The drawing under review shows one solid part. Ordinate dimensions are in mm from its lowest x, y, z. A direction names the side the tool comes from. Coordinates: 2 decimals unless noted, no trailing zeros. Write each loop counter-clockwise with the first axis right and the second up, starting at its lowest first coordinate (ties: lowest second). Pieces come first, ordered by that corner, then holes. Notation, with made-up numbers: (-30.75, -19.5) -> (25.25, -19.5) arc R12 cw to (25.25, -1.5) -> close; hole circle Ø10 at (26, 15). An arc over 180 degrees is marked (long way). One line per question, with ' | ' between items. Start each with the question number.
Q1. Add section C-C on z = 4.75. State the section outline as (x, y) points.
Q2. Wall thickness on probe 1 along X at (y, z) = (11, 5.55); probe 2 along X at (y, z) = (13, 1.9): over which ranges is each line inside the solid? List them lowest first.
Q3. For P1, Ø1.2, axis at x = 4.5, y = 24, coming from the +Z side; P2, Ø3, axis at y = 18, z = 4.5, coming from the +X side; P3, Ø2, axis at x = 2.5, y = 19, coming from the +Z side; P4, Ø1, axis at x = 1, y = 21, coming from the -Z side, all flat-tipped, find the tip position at first contact; note any pin that passes through.
Q4. Add section A-A on y = 31.5. State the section outline as (x, z) points, and give its area (3 significant figures).
Q5. For the marked faces 1 and 2, list the 3-axis set-ups (+Z, -Z, +X, -X, +Y, -Y) from which the entire face can be reached by the end or side of a thin tool; tool diameter is ignored.
Q6. Add section B-B on x = 5.5. State the section outline as (y, z) points.
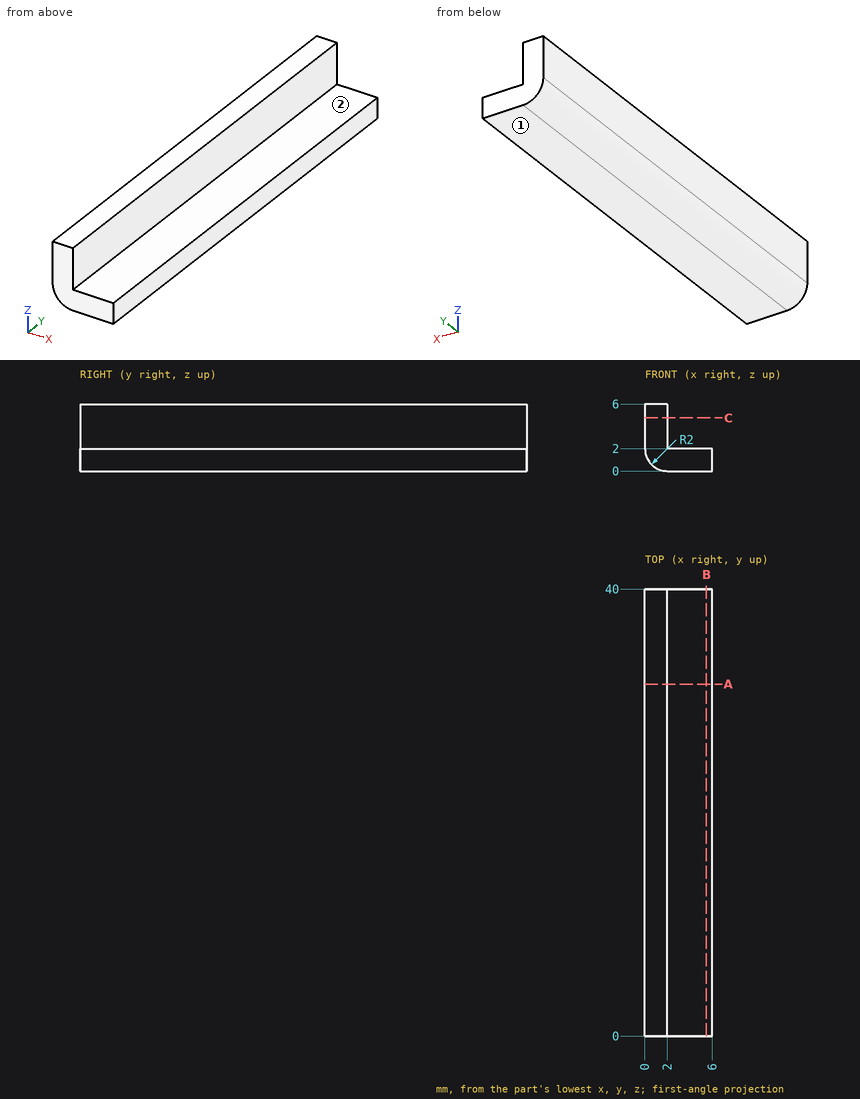
Output values:
1) outline: (0, 0) -> (2, 0) -> (2, 40) -> (0, 40) -> close
2) probe 1: x = 0 to 2 | probe 2: x = 0 to 6
3) P1: stops at z = 2 | P2: stops at x = 2 | P3: stops at z = 6 | P4: stops at z = 0.06
4) outline: (0, 2) arc R2 ccw to (2, 0) -> (6, 0) -> (6, 2) -> (2, 2) -> (2, 6) -> (0, 6) -> close | area: 19.1 mm2
5) face 1: -Z, +X, -X, +Y, -Y | face 2: +Z, +X, +Y, -Y
6) outline: (0, 0) -> (40, 0) -> (40, 2) -> (0, 2) -> close
